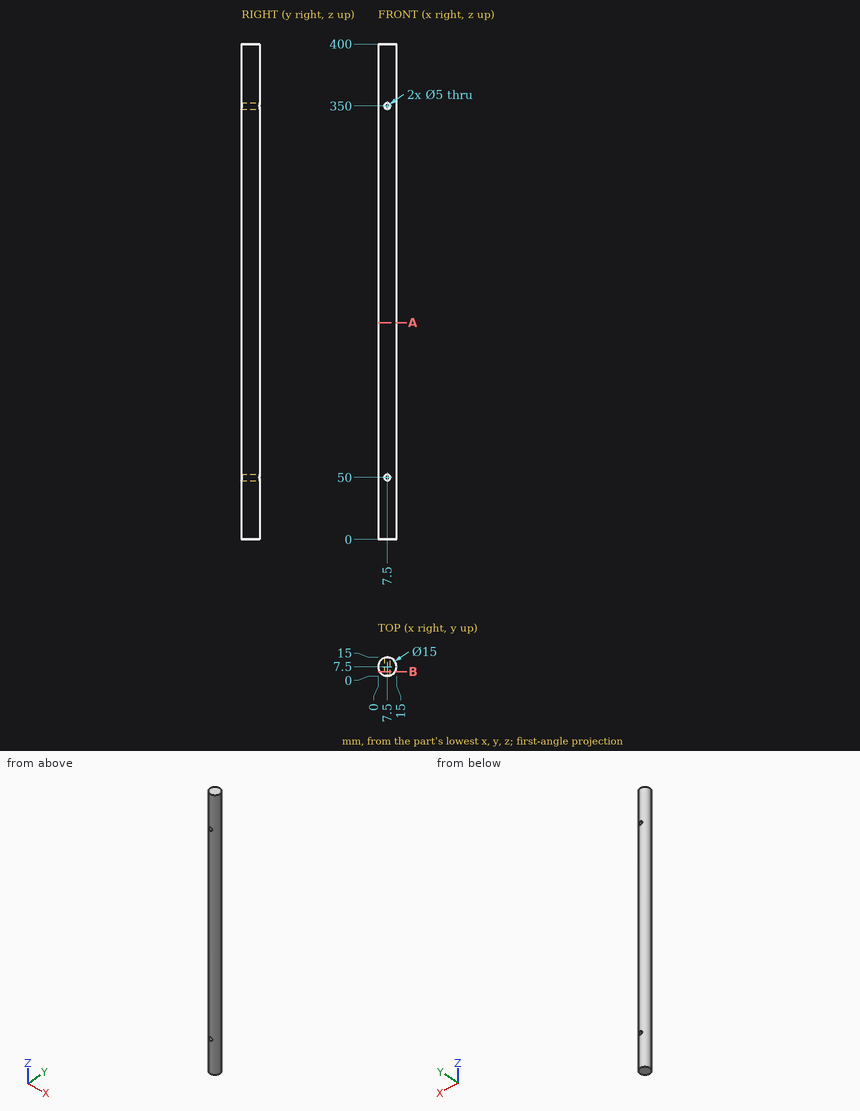
For this review, use the dimensioned drawing (mm, ordinates from the lowest corner) and the shaded views. Coordinates: 2 decimals unless noted, no trailing zeros. Write each loop counter-clockwise with the first axis right and the second up, starting at its lowest first coordinate (ties: lowest second). Pieces come first, ordered by that corner, then holes. Notation, with made-up numbers: (34, 32.25) - (78, 32.25) arc R21 cw to (78, 45.25) - close; hole circle Ø5 at (-37, 69.25). An arc over 180 degrees is marked (long way). Answer in a Markdown table with one row per item. Add a question column.
Q1. Clearance check with flat-ended pins moving along their axes: pin 1 (5 mm diameter, centred on y = 8, z = 93, fed in from +X); pin 2 (1.5 mm diameter, centred on x = 9.5, z = 287, fed in from +Y); pin 3 (4 mm diameter, centred on y = 4.5, z = 295.5, fed in from -X); pin 4 (1 mm diameter, centred on y = 11, z = 275, fed in from -X). State where each tip first meets the part, or that it passes through.
Q2. Consider section B-B on y = 3.5. Give the boundary of the cut face in (x, z).
Q3. To check wall thickness, follow line 1 along Z through (x, y) = (7.5, 11.5); line 2 along Z through (x, y) = (8.75, 3.5); line 3 along Y through (x, z) = (8.5, 44). State the ranges of each line that lie inside material, in increasing order. Write a range as from..to.
Q4. Consider section A-A on z = 175. Give the boundary of the cut face in (x, y).
Answers below:
| question | item | result |
|---|---|---|
| 1 | pin 1 | x = 15 |
| 1 | pin 2 | y = 14.9 |
| 1 | pin 3 | x = 0.07 |
| 1 | pin 4 | x = 0.63 |
| 2 | outline | (1.16, 0) - (13.84, 0) - (13.84, 400) - (1.16, 400) - close; hole circle Ø5 at (7.5, 50); hole circle Ø5 at (7.5, 350) |
| 3 | line 1 | 0..47.5, 52.5..347.5, 352.5..400 |
| 3 | line 2 | 0..47.83, 52.17..347.83, 352.17..400 |
| 3 | line 3 | 0.07..14.93 |
| 4 | outline | circle Ø15 at (7.5, 7.5) |
